Geometry check sheet. Reference: drawing and pictorial views, mm from the part's lowest x, y, z. A direction names the side the tool comes from. Round coordinates to 2 decimals unless told otherwise and drop trailing zeros. Loops run counter-clockwise (first coordinate to the right, second up) from the corner with the lowest first, then second, coordinate; pieces in that order, holes last. Notation, with made-up numbers: (13.25, 87) - (45.25, 87) arc R3 ccw to (45.25, 92) - close; hole circle Ø7 at (32.25, -34.75). An arc over 180 degrees is marked (long way). Put each result on its own line as item: value. Start each with the question number.
Item 1: Material ranges on line 1 along X through (y, z) = (62.5, 41) (1 decimal); line 2 along Y through (x, z) = (105, 48) (1 decimal); line 3 along X through (y, z) = (115.5, 61.5) (1 decimal), recorded low to high.
Item 2: Section check A-A, the plane z = 64.5. Record the cut outline in (x, y) (1 decimal), and give its area (3 significant figures).
Item 3: Draft check along Y on the marked faces 1, 2 and 3. Enter one of: pulls with the +Y half, pulls with the -Y half, needs draft (parallel to the pull), parting line crosses it, or undercut.
Item 4: Gauge pin test, flat ends, axial feed: pin 1 Ø1 at (y, z) = (93.5, 46) entering from -X; pin 2 Ø5 at (x, z) = (46.5, 31) entering from -Y; pin 3 Ø12 at (x, y) = (51, 71.5) entering from +Z; pin 4 Ø1.5 at (x, z) = (15.5, 54) entering from +Y. Record the tip position at first contact, or that the pin passes through.
Item 5: Section check B-B, the plane y = 60.5. Record the cut outline in (x, z) (1 decimal), and give its area (3 significant figures).
Item 6: Section check D-D, the plane x = 9. Record the cut outline in (y, z), and give its area (3 significant figures).
Item 7: Section check C-C, the plane z = 41. Record the cut outline in (x, y), and give its area (3 significant figures).
Item 8: Tool access check on the marked faces 4, 5 and 6. Record the directions out of +Z, -Z, +X, -X, +Y, -Y that give a thin tool (end or side, any length) a straight path to the whole face; none if there is none.
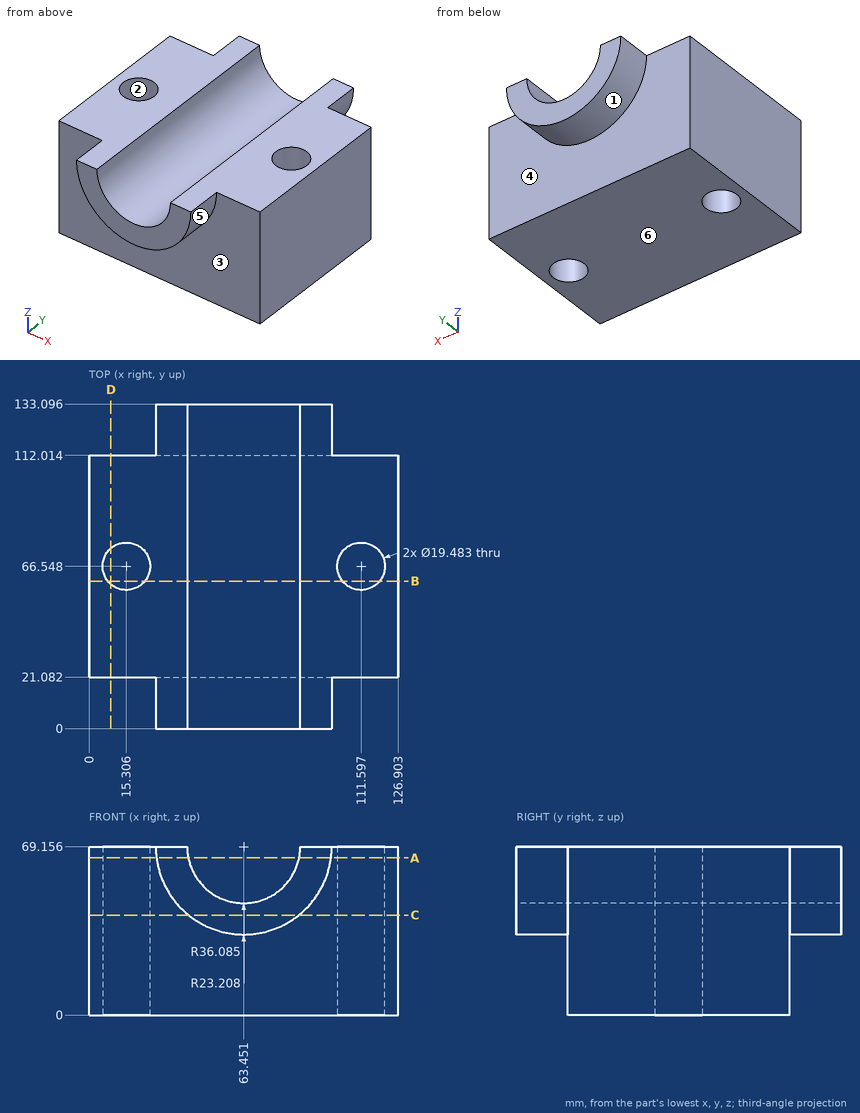
Check result:
1. line 1: 0 to 6.4, 24.2 to 102.7, 120.5 to 126.9
1. line 2: 21.1 to 59.4, 73.7 to 112
1. line 3: 28.2 to 41.5, 85.4 to 98.7
2. outline: (0, 21.1) - (27.7, 21.1) - (27.7, 0) - (40.7, 0) - (40.7, 133.1) - (27.7, 133.1) - (27.7, 112) - (0, 112) - close; (86.2, 0) - (99.2, 0) - (99.2, 21.1) - (126.9, 21.1) - (126.9, 112) - (99.2, 112) - (99.2, 133.1) - (86.2, 133.1) - close; hole circle Ø19.5 at (15.3, 66.5); hole circle Ø19.5 at (111.6, 66.5)
2. area: 7,910 mm²
3. face 1: needs draft
3. face 2: undercut
3. face 3: pulls with the -Y half
4. pin 1: x = 0
4. pin 2: y = 21.08
4. pin 3: z = 55.08
4. pin 4: y = 112.01
5. outline: (0, 0) - (7.7, 0) - (7.7, 69.2) - (0, 69.2) - close; (22.9, 0) - (104, 0) - (104, 69.2) - (86.7, 69.2) arc R23.2 cw to (40.2, 69.2) - (22.9, 69.2) - close; (119.2, 0) - (126.9, 0) - (126.9, 69.2) - (119.2, 69.2) - close
5. area: 5,820 mm²
6. outline: (21.08, 0) - (59.12, 0) - (59.12, 69.16) - (21.08, 69.16) - close; (73.97, 0) - (112.01, 0) - (112.01, 69.16) - (73.97, 69.16) - close
6. area: 5,260 mm²
7. outline: (0, 21.08) - (40.88, 21.08) - (40.88, 0) - (86.02, 0) - (86.02, 21.08) - (126.9, 21.08) - (126.9, 112.01) - (86.02, 112.01) - (86.02, 133.1) - (40.88, 133.1) - (40.88, 112.01) - (0, 112.01) - close; hole circle Ø19.48 at (15.31, 66.55); hole circle Ø19.48 at (111.6, 66.55)
7. area: 12,800 mm²
8. face 4: -Z, +Y
8. face 5: -Z, -Y
8. face 6: -Z, +X, -X, +Y, -Y
